Check sheet for the modelled part. Datum: model origin and axes. Units: mm. A direction names the side the tool comes from. Coordinates: 2 decimals unless noted, no trailing zeros. Loops run counter-clockwise (first coordinate to the right, second up) from the corner with the lowest first, then second, coordinate; pieces in that order, holes last. Notation, with made-up numbers: (-22, 20.5) - (-13, 20.5) arc R22 cw to (-13, 50.5) - close; hole circle Ø9 at (39.5, -1.5). An arc over 180 degrees is marked (long way). Use a Markdown table: item, result. Add a question column.
1) Sectioned sample at A-A, the plane y = 15. Enter the section's corners in (x, z), then the cut area to 3 significant figures.
2) Sectioned sample at C-C, the plane z = 7.25. Enter the section's corners in (x, y).
3) Sectioned sample at B-B, the plane x = -100. Enter the section's corners in (y, z), then the cut area to 3 significant figures.
4) Sectioned sample at D-D, the plane y = -25. Enter the section's corners in (x, z).
5) Draft check along Y on faces 1 (the flat face through (-2, -46.5, 5)), 2 (the flat face through (120, -1, 5)), 3 (the cylindrical face through (72.753, 15.143, 2.028)). Enter one of: pulls with the +Y half, pulls with the -Y half, needs draft (parallel to the pull), parting line crosses it, or undercut.
6) Tool access check on faces 4 (the cylindrical face through (81, 16.6, 7.5)), 5 (the cylindrical face through (-26.395, 17.197, 2.028)). Record the directions out of +Z, -Z, +X, -X, +Y, -Y that give a thin tool (end or side, any length) a straight path to the whole face; none if there is none.
7) Go/stop test with flat-tipped pins: P1, Ø12, axis at x = -18, y = -2, coming from the -Z side; P2, Ø4, axis at x = -24, y = -15, coming from the +Z side; P3, Ø8.5, axis at x = -24, y = -15.5, coming from the +Z side. Record where each tip stops, or that it passes through.
8) Thickness scan on line 1 (Y direction, x = 76, z = 2.2); line 2 (Y direction, x = -24, z = 7.25). Record the ranges inside material, lowest first.
from build123d import *

# Parameters (mm, degrees)
F0_W     = 240
F0_H     = 93
F1_DEPTH = 11
F2_R     = 3.25
F2_R_2   = 3
F3_DEPTH = 11.001
F4_R     = 5.25
F5_DEPTH = 7


with BuildPart() as f1:
    # F0 (on Top) → F1 (new body)
    with BuildSketch(Plane.XY):
        Rectangle(F0_W, F0_H)
    extrude(amount=F1_DEPTH)

    # F2 (on face) → F3 (cut, through all)
    with BuildSketch(Plane.XY.offset(11)):
        with Locations((76, 15)):
            Circle(F2_R)
        with Locations((-24, 15)):
            Circle(F2_R)
        with Locations((-100, 25)):
            Circle(F2_R_2)
        with Locations((-100, -25)):
            Circle(F2_R_2)
        with Locations((-24, -15)):
            Circle(F2_R)
        with Locations((76, -15)):
            Circle(F2_R)
    extrude(amount=-F3_DEPTH, mode=Mode.SUBTRACT)

    # F4 (on face) → F5 (cut)
    with BuildSketch(Plane.XY.offset(11)):
        with Locations((-24, 15)):
            Circle(F4_R)
        with Locations((76, 15)):
            Circle(F4_R)
        with Locations((76, -15)):
            Circle(F4_R)
        with Locations((-24, -15)):
            Circle(F4_R)
    extrude(amount=-F5_DEPTH, mode=Mode.SUBTRACT)


solid = f1.part
Solved:
| question | item | result |
|---|---|---|
| 1 | outline | (-120, 0) - (-27.25, 0) - (-27.25, 4) - (-29.25, 4) - (-29.25, 11) - (-120, 11) - close; (-20.75, 0) - (72.75, 0) - (72.75, 4) - (70.75, 4) - (70.75, 11) - (-18.75, 11) - (-18.75, 4) - (-20.75, 4) - close; (79.25, 0) - (120, 0) - (120, 11) - (81.25, 11) - (81.25, 4) - (79.25, 4) - close |
| 1 | area | 2,440 mm2 |
| 2 | outline | (-120, -46.5) - (120, -46.5) - (120, 46.5) - (-120, 46.5) - close; hole circle Ø6 at (-100, -25); hole circle Ø6 at (-100, 25); hole circle Ø10.5 at (-24, -15); hole circle Ø10.5 at (-24, 15); hole circle Ø10.5 at (76, -15); hole circle Ø10.5 at (76, 15) |
| 3 | outline | (-46.5, 0) - (-28, 0) - (-28, 11) - (-46.5, 11) - close; (-22, 0) - (22, 0) - (22, 11) - (-22, 11) - close; (28, 0) - (46.5, 0) - (46.5, 11) - (28, 11) - close |
| 3 | area | 891 mm2 |
| 4 | outline | (-120, 0) - (-103, 0) - (-103, 11) - (-120, 11) - close; (-97, 0) - (120, 0) - (120, 11) - (-97, 11) - close |
| 5 | face 1 | pulls with the -Y half |
| 5 | face 2 | needs draft |
| 5 | face 3 | undercut |
| 6 | face 4 | +Z |
| 6 | face 5 | +Z, -Z |
| 7 | P1 | stops at z = 0 |
| 7 | P2 | passes through |
| 7 | P3 | stops at z = 4 |
| 8 | line 1 | y = -46.5 to -18.25, -11.75 to 11.75, 18.25 to 46.5 |
| 8 | line 2 | y = -46.5 to -20.25, -9.75 to 9.75, 20.25 to 46.5 |
